Geometry: final body of the model. Coordinates: model frame, mm. Give positions to 0.01 mm unless a question says otherwise; leave off trailing zeros. Write each loop counter-clockwise with the first axis right and the second up, starting at its lowest first coordinate (ties: lowest second). Pieces come first, ordered by that corner, then holes.
Q1. Cut plane A-A on y = 4.25. Count the separate pieces of the cut face and the enclosed holes in it, plus the area to 3 significant figures.
Q2. Line query: L1, parallel to X at y = 13.25, z = -34.5; L2, parallel to Z at x = -182, y = 2.5; L3, parallel to X at y = 6.5, z = -36. Output: solid intervals per line, ascending.
Q3. Cut plane C-C on z = -165. Return the cut outline in (x, y).
Q4. Pin query (flat end, axial travel): pin 1 (3 mm diameter, centred on y = 12, z = -127, fed in from -X); pin 2 (6 mm diameter, centred on x = 716.5, y = 5, fed in from +Z); pin 3 (4.5 mm diameter, centred on x = -120.49, z = -75.37, fed in from +Y); pin 4 (3 mm diameter, centred on x = -71, y = 2, fed in from -Z). Return the tip coordinate at first contact, or that it passes through.
Q5. Cut plane B-B on x = 813.5. Return the cut outline in (y, z).
```python
from build123d import *

# Parameters (mm, degrees)
BOSS_EXTRUDE1_DEPTH = 15.24
SKETCH2_R           = 2.38125
CUT_EXTRUDE1_DEPTH  = 15.24
CHAMFER1_SIZE       = 8.89


with BuildPart() as part:
    # Sketch1 → Boss-Extrude1 (new body)
    with BuildSketch(Plane(origin=(0, 0, 0), x_dir=(1, 0, 0), z_dir=(0, 1, 0))):
        Polygon((-241.141854356, 15.046517442), (-241.141854356, 94.421517442), (-203.041854356, 108.709017442), (-50.641854356, 108.709017442), (114.335985065, 203.959017442), (368.335985065, 203.959017442), (622.335985065, 203.959017442), (787.313824486, 108.709017442), (939.713824486, 108.709017442), (977.813824486, 94.421517442), (977.813824486, 15.046517442), (939.713824486, 0.759017442), (787.313824486, 0.759017442), (622.335985065, -94.490982558), (368.335985065, -94.490982558), (114.335985065, -94.490982558), (-50.641854356, 0.759017442), (-203.041854356, 0.759017442), align=None)
    extrude(amount=BOSS_EXTRUDE1_DEPTH)

    # Sketch2 → Cut-Extrude1 (cut)
    with BuildSketch(Plane(origin=(0, 0, 0), x_dir=(-1, 0, 0), z_dir=(0, -1, 0))):
        with Locations(Location((183.991854356, 34.096517442, 0), (0, 0, 90))):
            Circle(SKETCH2_R)
        with Locations(Location((183.991854356, 75.371517443, 0), (0, 0, 90))):
            Circle(SKETCH2_R)
        with Locations(Location((120.491854356, 75.371517443, 0), (0, 0, 90))):
            Circle(SKETCH2_R)
        with Locations(Location((120.491854356, 34.096517443, 0), (0, 0, 90))):
            Circle(SKETCH2_R)
        with Locations(Location((-857.163824486, 75.371517443, 0), (0, 0, 90))):
            Circle(SKETCH2_R)
        with Locations(Location((-920.663824486, 75.371517443, 0), (0, 0, 90))):
            Circle(SKETCH2_R)
        with Locations(Location((-920.663824486, 34.096517442, 0), (0, 0, 90))):
            Circle(SKETCH2_R)
        with Locations(Location((-857.163824486, 34.096517443, 0), (0, 0, 90))):
            Circle(SKETCH2_R)
    extrude(amount=-CUT_EXTRUDE1_DEPTH, mode=Mode.SUBTRACT)

    # Chamfer1
    chamfer1_edges = [part.edges().sort_by_distance(p)[0] for p in [
        (-126.841854356, 0, -0.759017442),
        (-222.091854356, 0, -7.902767442),
        (-241.141854356, 0, -54.734017442),
        (-222.091854356, 0, -101.565267442),
        (-126.841854356, 0, -108.709017442),
        (31.847065354, 0, -156.334017442),
        (368.335985065, 0, -203.959017442),
        (704.824904775, 0, -156.334017442),
        (863.513824486, 0, -108.709017442),
        (958.763824486, 0, -101.565267442),
        (977.813824486, 0, -54.734017442),
        (958.763824486, 0, -7.902767442),
        (863.513824486, 0, -0.759017442),
        (704.824904775, 0, 46.865982558),
        (368.335985065, 0, 94.490982558),
        (31.847065354, 0, 46.865982558),
    ]]
    chamfer(chamfer1_edges, length=CHAMFER1_SIZE)


solid = part.part
```
Data:
1. separate pieces: 1
1. enclosed holes: 8
1. area: 246,000 mm2
2. L1: x = -241.14 to -186.34, -181.65 to -122.84, -118.15 to 854.82, 859.51 to 918.32, 923.01 to 977.81
2. L2: z = -102.32 to -76.68, -74.07 to -35.4, -32.79 to -7.15
2. L3: x = -238.75 to -185.42, -182.56 to -121.92, -119.06 to 855.73, 858.59 to 919.23, 922.09 to 975.42
3. outline: (46.86, 8.89) - (64.64, 0) - (672.03, 0) - (689.81, 8.89) - (689.81, 15.24) - (46.86, 15.24) - close
4. pin 1: stops at x = -21.56
4. pin 2: stops at z = 39.51
4. pin 3: passes through
4. pin 4: stops at z = -103.32
5. outline: (0, -99.82) - (8.89, -108.71) - (15.24, -108.71) - (15.24, -0.76) - (8.89, -0.76) - (0, -9.65) - close
